```python
from build123d import *

# Parameters (mm, degrees)
SKETCH_1_R               = 6
EXTRUDE_1_DEPTH          = 4.5
SKETCH_3_R               = 6
SKETCH_3_R_2             = 5.5
EXTRUDE_2_DEPTH          = 1
CUT_EXTRUDE_3_DEPTH      = 39.003289331
CUT_EXTRUDE_3_DEPTH_BACK = 39.003289331
SKETCH_5_R               = 1.5
SKETCH_6_R               = 1.5
CUT_EXTRUDE_4_DEPTH      = 5


with BuildPart() as part:
    # 草图1 → 凸台-拉伸1 (new body)
    with BuildSketch(Plane.XY):
        with BuildLine():
            Line((-20, 0), (-20, -32))
            Line((-20, -32), (20, -32))
            Line((20, -32), (20, 0))
            ThreePointArc((20, 0), (0, 20), (-20, 0))
        make_face()
        Circle(SKETCH_1_R, mode=Mode.SUBTRACT)
    extrude(amount=EXTRUDE_1_DEPTH)

    # 草图3 → 凸台-拉伸2 (add)
    with BuildSketch(Plane.XY):
        Circle(SKETCH_3_R)
        Circle(SKETCH_3_R_2, mode=Mode.SUBTRACT)
    extrude(amount=EXTRUDE_2_DEPTH)

    # 草图5 → 切除-拉伸3 (cut, two sides: drawn at the far end of the back side and taken through both)
    with BuildSketch(Plane.XY.offset(-CUT_EXTRUDE_3_DEPTH_BACK)):
        with Locations((0, 16)):
            Circle(SKETCH_5_R)
        with Locations((-16, 0)):
            Circle(SKETCH_5_R)
        with Locations((16, 0)):
            Circle(SKETCH_5_R)
    extrude(amount=CUT_EXTRUDE_3_DEPTH + CUT_EXTRUDE_3_DEPTH_BACK, mode=Mode.SUBTRACT)

    # 草图6 → 切除-拉伸4 (cut)
    with BuildSketch(Plane.XZ.offset(32)):
        with Locations(Location((9, 2.25, 0), (0, 0, 270))):
            Circle(SKETCH_6_R)
        with Locations(Location((-9, 2.25, 0), (0, 0, 270))):
            Circle(SKETCH_6_R)
    extrude(amount=-CUT_EXTRUDE_4_DEPTH, mode=Mode.SUBTRACT)


solid = part.part
```
Read the model definition and answer for the solid it produces. Units are mm, in the model's axes. A direction names the side the tool comes from. Coordinates: 2 decimals unless noted, no trailing zeros. Write each loop counter-clockwise with the first axis right and the second up, starting at its lowest first coordinate (ties: lowest second). Pieces come first, ordered by that corner, then holes. Notation, with made-up numbers: (4.25, 62) - (26.25, 62) arc R17 cw to (26.25, 66) - close; hole circle Ø11 at (65.5, 80.5). An arc over 180 degrees is marked (long way). Answer as a JSON object with one key per item and string values. Group by question number.
1. Each of these flat-tipped pins is pushed along its axis until it touches: P1, Ø9, axis at x = 0, y = 0, coming from the +Z side; P2, Ø1.5, axis at x = -9, z = 2, coming from the -Y side. Where does it stop, or does it pass through?
2. The mould has two halves that part along X. Classify faces 4 (the flat face through (-9, -27, 2)), 5 (the flat face through (20, -16, 2)), 6 (the flat face through (-20, -16, 2)): +X half, -X half, draft (parallel to the pull), parting line (faces both ways), or undercut.
3. A cutting plane is placed at B-B (z = 2.25). Determine the outline of the cut face in (x, y), plus the area to 3 significant figures.
4. Which of the six approach directions +Z, -Z, +X, -X, +Y, -Y give full straight-line access (tool end or side, diameter ignored) to faces 1 (the cylindrical face through (-6, 0, 3)), 2 (the cylindrical face through (7.67, -29.54, 1.56)), 3 (the cylindrical face through (-1.19, -5.37, 0.49))?
5. A cutting plane is placed at A-A (x = 16). Determine the outline of the cut face in (y, z).
6. A cutting plane is placed at C-C (x = -16.5). Determine the outline of the cut face in (y, z), plus the area to 3 significant figures.
7. Consider L1, parallel to Y at x = 0, z = 2.8; L2, parallel to X at y = -28.65, z = 2.25; L3, parallel to Y at x = 0, z = 0.35. Determine where each line is inside the solid, lowest interval first. Write a range as [from, to].
8. A cutting plane is placed at D-D (x = -9). Determine the outline of the cut face in (y, z).
Worked out:
{
 "1": {"P1": "passes through", "P2": "stops at y = -27"},
 "2": {"face 4": "undercut", "face 5": "+X half", "face 6": "-X half"},
 "3": {"outline": "(-20, -32) - (-10.5, -32) - (-10.5, -27) - (-7.5, -27) - (-7.5, -32) - (7.5, -32) - (7.5, -27) - (10.5, -27) - (10.5, -32) - (20, -32) - (20, 0) arc R20 ccw to (-20, 0) - close; hole circle Ø3 at (-16, 0); hole circle Ø12 at (0, 0); hole circle Ø3 at (0, 16); hole circle Ø3 at (16, 0)", "area": "1,740 mm²"},
 "4": {"face 1": "+Z", "face 2": "-Y", "face 3": "+Z, -Z"},
 "5": {"outline": "(-32, 0) - (-1.5, 0) - (-1.5, 4.5) - (-32, 4.5) - close; (1.5, 0) - (12, 0) - (12, 4.5) - (1.5, 4.5) - close"},
 "6": {"outline": "(-32, 0) - (-1.41, 0) - (-1.41, 4.5) - (-32, 4.5) - close; (1.41, 0) - (11.3, 0) - (11.3, 4.5) - (1.41, 4.5) - close", "area": "182 mm²"},
 "7": {"L1": "y = [-32, -6], [6, 14.5], [17.5, 20]", "L2": "x = [-20, -10.5], [-7.5, 7.5], [10.5, 20]", "L3": "y = [-32, -5.5], [5.5, 14.5], [17.5, 20]"},
 "8": {"outline": "(-32, 0) - (17.86, 0) - (17.86, 4.5) - (-32, 4.5) - (-32, 3.75) - (-27, 3.75) - (-27, 0.75) - (-32, 0.75) - close"}
}
